Geometry check sheet. Reference: the model listing, model coordinates, mm. Face numbers are marked on the shaded views. Give positions to 0.01 mm unless a question says otherwise; leave off trailing zeros. Write each loop counter-clockwise with the first axis right and the second up, starting at its lowest first coordinate (ties: lowest second). Pieces come first, ordered by that corner, then holes. Notation, with made-up numbers: (-5, -20) -> (0, -20) arc R20 ccw to (0, -8) -> close; hole circle Ø7 at (60, 26.5). An arc over 180 degrees is marked (long way). Use a Markdown table: item, result. Add a question column.
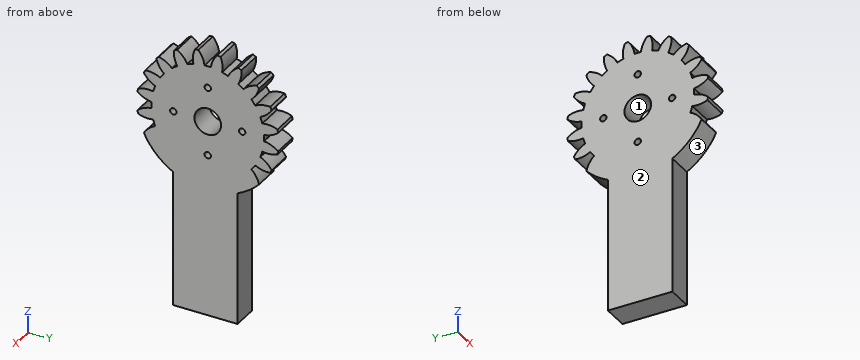
from build123d import *

# Parameters (mm, degrees)
BASPROSKE_W             = 6
BASPROSKE_H             = 16.5
TOOTHCUT_DEPTH          = 25.093567606
TEETHCUTS_COUNT         = 20
TEETHCUTS_ANGLE         = 342
BORSKE_R                = 3.1
BORE_DEPTH              = 50.0000508
ESQUISSE2_W             = 34.6
ESQUISSE2_H             = 15
BOSS_EXTRU_1_DEPTH      = 6
ESQUISSE3_R             = 0.75
ENL_V_MAT_EXTRU_1_DEPTH = 6


with BuildPart() as part:
    # BasProSke → Base-Revolve (revolve)
    with BuildSketch(Plane(origin=(0, 0, 0), x_dir=(1, 0, 0), z_dir=(0, 1, 0)), mode=Mode.PRIVATE) as base_revolve_sk:
        with Locations((3, 8.25)):
            Rectangle(BASPROSKE_W, BASPROSKE_H)
    revolve(base_revolve_sk.sketch.rotate(Axis((-10, 0, 0), (1, 0, 0)), 180), axis=Axis((-10, 0, 0), (1, 0, 0)))

    # TooCutSke → ToothCut (cut, through all)
    with BuildSketch(Plane(origin=(0, 0, 0), x_dir=(0, 0, -1), z_dir=(1, 0, 0))):
        with BuildLine():
            ThreePointArc((0.74381438, 13.102904875), (0, 13.124), (-0.74381438, 13.102904875))
            ThreePointArc((-0.74381438, 13.102904875), (-1.226473103, 14.852072512), (-2.209965745, 16.376962373))
            ThreePointArc((-2.209965745, 16.376962373), (0, 16.5254), (2.209965745, 16.376962373))
            ThreePointArc((2.209965745, 16.376962373), (1.226473103, 14.852072512), (0.74381438, 13.102904875))
        make_face()
    toothcut = extrude(amount=TOOTHCUT_DEPTH, mode=Mode.SUBTRACT)

    # TeethCuts: ToothCut ×20 about axis, 6 skipped
    teethcuts_axis = Axis((-10, 0, 0), (1, 0, 0))
    add([toothcut.rotate(teethcuts_axis, i * TEETHCUTS_ANGLE / (TEETHCUTS_COUNT - 1)) for i in range(1, TEETHCUTS_COUNT) if i not in (12, 13, 14, 15, 16, 17)], mode=Mode.SUBTRACT)

    # BorSke → Bore (cut, symmetric)
    with BuildSketch(Plane(origin=(0, 0, 0), x_dir=(0, 0, -1), z_dir=(1, 0, 0))):
        with Locations(Location((0, 0, 0), (0, 0, 180))):
            Circle(BORSKE_R)
    extrude(amount=BORE_DEPTH, both=True, mode=Mode.SUBTRACT)

    # Esquisse2 → Boss.-Extru.1 (add)
    with BuildSketch(Plane(origin=(6, 0, 0), x_dir=(0, 0, -1), z_dir=(1, 0, 0))):
        with Locations((28.717803782, -0.556420359)):
            Rectangle(ESQUISSE2_W, ESQUISSE2_H)
    extrude(amount=-BOSS_EXTRU_1_DEPTH)

    # Esquisse3 → Enlèv. mat.-Extru.1 (cut)
    with BuildSketch(Plane.ZY):
        with Locations((8, 0)):
            Circle(ESQUISSE3_R)
        with Locations((0, 8)):
            Circle(ESQUISSE3_R)
        with Locations((0, -8)):
            Circle(ESQUISSE3_R)
        with Locations((-8, 0)):
            Circle(ESQUISSE3_R)
    extrude(amount=-ENL_V_MAT_EXTRU_1_DEPTH, mode=Mode.SUBTRACT)


solid = part.part
1) Draft check along Y on the marked faces 1, 2 and 3. Enter one of: +Y half, -Y half, draft (parallel to the pull), parting line (faces both ways), or undercut.
2) Sectioned sample at D-D, the plane y = 6. Enter the section's corners in (x, z), and give its area (3 significant figures).
3) Sectioned sample at A-A, the plane y = 0. Enter the section's corners in (x, z).
4) Sectioned sample at B-B, the plane z = -26.5. Enter the section's corners in (x, y).
5) Gauge pin test, flat ends, axial feed: P1, Ø1.8, axis at x = 2, z = -24, coming from the +Y side; P2, Ø1.2, axis at y = 0, z = -8, coming from the +X side; P3, Ø1, axis at x = 1.5, y = 1.5, coming from the +Z side. Record the tip position at first contact, or that the pin passes through.
6) Material ranges on probe 1 along Y at (x, z) = (3.95, 0); probe 2 along Y at (x, z) = (3.85, 0.5); probe 3 along Y at (x, z) = (3.5, -5), recorded low to high. Write a range as [from, to].
7) Sectioned sample at C-C, the plane x = 2.05. Count the separate pieces of the cut face and the enclosed holes in it, and give its area (3 significant figures).
Check values:
| question | item | result |
|---|---|---|
| 1 | face 1 | undercut |
| 1 | face 2 | draft |
| 1 | face 3 | -Y half |
| 2 | outline | (0, -46.02) -> (6, -46.02) -> (6, 14) -> (0, 14) -> close |
| 2 | area | 360 mm² |
| 3 | outline | (0, -46.02) -> (6, -46.02) -> (6, -8.75) -> (0, -8.75) -> close; (0, -7.25) -> (6, -7.25) -> (6, -3.1) -> (0, -3.1) -> close; (0, 3.1) -> (6, 3.1) -> (6, 7.25) -> (0, 7.25) -> close; (0, 8.75) -> (6, 8.75) -> (6, 13.12) -> (0, 13.12) -> close |
| 4 | outline | (0, -8.06) -> (6, -8.06) -> (6, 6.94) -> (0, 6.94) -> close |
| 5 | P1 | y = 6.94 |
| 5 | P2 | through |
| 5 | P3 | z = 16.13 |
| 6 | probe 1 | [-13.12, -8.75], [-7.25, -3.1], [3.1, 7.25], [8.75, 13.12] |
| 6 | probe 2 | [-13.11, -8.56], [-7.44, -3.06], [3.06, 7.44], [8.56, 13.11] |
| 6 | probe 3 | [-12.7, 12.7] |
| 7 | separate pieces | 1 |
| 7 | enclosed holes | 5 |
| 7 | area | 1,150 mm² |
